from build123d import *

# Parameters (mm, degrees)
F1_DEPTH        = 25
F3_START        = -0.65
F2_R            = 4.3
F3_DEPTH        = 2.15
F3_COPIES_COUNT = 3
F6_DEPTH        = 23
F8_DEPTH        = 2
F9_SIZE         = 0.6
F10_SIZE        = 0.4


# Not quite as in the source:
# - a pattern or mirror of a feature is missing from the dataset's text; its kind, count and spacing are read off the source's solid


with BuildPart() as f1:
    # F0 (on Top) → F1 (new body)
    with BuildSketch(Plane.XY):
        with BuildLine():
            ThreePointArc((7.6794919243, -4), (19.8038475773, 3), (19.8038475773, 17))
            Line((19.8038475773, 17), (12.124355653, 30.3012701892))
            ThreePointArc((12.124355653, 30.3012701892), (0, 37.3012701892), (-12.124355653, 30.3012701892))
            Line((-12.124355653, 30.3012701892), (-19.8038475773, 17))
            ThreePointArc((-19.8038475773, 17), (-19.8038475773, 3), (-7.6794919243, -4))
            Line((-7.6794919243, -4), (0, -4))
            Line((0, -4), (7.6794919243, -4))
        make_face()
        with BuildLine():
            Line((7.6794919243, 0), (0, 0))
            Line((0, 0), (-7.6794919243, 0))
            ThreePointArc((-7.6794919243, 0), (-16.3397459622, 5), (-16.3397459622, 15))
            Line((-16.3397459622, 15), (-8.6602540378, 28.3012701892))
            ThreePointArc((-8.6602540378, 28.3012701892), (0, 33.3012701892), (8.6602540378, 28.3012701892))
            Line((8.6602540378, 28.3012701892), (16.3397459622, 15))
            ThreePointArc((16.3397459622, 15), (16.3397459622, 5), (7.6794919243, 0))
        make_face(mode=Mode.SUBTRACT)
    extrude(amount=F1_DEPTH)

    # F2 (on face) → F3 (cut)
    with BuildSketch(Plane(origin=(-22.2141016151, 12.8253175473, 0), x_dir=(-0.5, -0.8660254038, 0), z_dir=(-0.8660254038, 0.5, 0)).offset(F3_START)):
        with Locations((-12.5, 12.5)):
            Circle(F2_R)
    f3 = extrude(amount=-F3_DEPTH, mode=Mode.SUBTRACT)

    # F3_copies: F3 ×3 about axis
    f3_copies_axis = Axis((0, 14.433757, 0), (0, 0, 1))
    for i in range(1, F3_COPIES_COUNT):
        add(f3.rotate(f3_copies_axis, i * 360 / F3_COPIES_COUNT), mode=Mode.SUBTRACT)

    # F5 (on face) → F6 (cut)
    with BuildSketch(Plane(origin=(0, 0, 0), x_dir=(1, 0, 0), z_dir=(0, 0, -1))):
        with BuildLine():
            Line((9.6994845224, -28.9012701892), (17.3789764467, -15.6))
            ThreePointArc((17.3789764467, -15.6), (17.3789764467, -4.4), (7.6794919243, 1.2))
            Line((7.6794919243, 1.2), (-7.6794919243, 1.2))
            ThreePointArc((-7.6794919243, 1.2), (-17.3789764467, -4.4), (-17.3789764467, -15.6))
            Line((-17.3789764467, -15.6), (-9.6994845224, -28.9012701892))
            ThreePointArc((-9.6994845224, -28.9012701892), (0, -34.5012701892), (9.6994845224, -28.9012701892))
        make_face()
    extrude(amount=-F6_DEPTH, mode=Mode.SUBTRACT)

    # F7 (on face) → F8 (cut)
    with BuildSketch(Plane(origin=(0, 0, 0), x_dir=(1, 0, 0), z_dir=(0, 0, -1))):
        with BuildLine():
            Line((11.0851251684, -29.7012701892), (18.7646170928, -16.4))
            ThreePointArc((18.7646170928, -16.4), (18.7646170928, -3.6), (7.6794919243, 2.8))
            Line((7.6794919243, 2.8), (-7.6794919243, 2.8))
            ThreePointArc((-7.6794919243, 2.8), (-18.7646170928, -3.6), (-18.7646170928, -16.4))
            Line((-18.7646170928, -16.4), (-11.0851251684, -29.7012701892))
            ThreePointArc((-11.0851251684, -29.7012701892), (0, -36.1012701892), (11.0851251684, -29.7012701892))
        make_face()
    extrude(amount=-F8_DEPTH, mode=Mode.SUBTRACT)

    # F9
    f9_edges = [f1.edges().sort_by_distance(p)[0] for p in [
        (0, 34.50127, 2),
        (13.53923, 22.250635, 2),
        (17.378976, 4.4, 2),
        (0, -1.2, 2),
        (-17.378976, 4.4, 2),
        (-13.53923, 22.250635, 2),
    ]]
    chamfer(f9_edges, length=F9_SIZE)

    # F10
    f10_edges = [f1.edges().sort_by_distance(p)[0] for p in [
        (19.803848, 3, 25),
        (12.5, 21.650635, 25),
        (0, -4, 25),
        (-19.803848, 3, 25),
        (-15.964102, 23.650635, 25),
        (15.964102, 23.650635, 25),
        (0, 37.30127, 25),
        (16.339746, 5, 25),
        (0, 0, 25),
        (-16.339746, 5, 25),
        (-12.5, 21.650635, 25),
        (0, 33.30127, 25),
    ]]
    chamfer(f10_edges, length=F10_SIZE)


solid = f1.part
Check sheet for the modelled part. Datum: model origin and axes. Units: mm. A direction names the side the tool comes from. Coordinates: 2 decimals unless noted, no trailing zeros. Write each loop counter-clockwise with the first axis right and the second up, starting at its lowest first coordinate (ties: lowest second). Pieces come first, ordered by that corner, then holes. Notation, with made-up numbers: M 58,-0.5 L 90,-0.5 A16 cw 90,6.5 Z; hole C -38,35 d11. An arc over 180 degrees is marked long. Answer as CSV lines item,"result".
Q1. Cross-section at D-D (z = 11.75). Record the boundary of the cut face in (x, y), then the cut area to 3 significant figures.
Check result:
outline,"M -19.8,17 A14 ccw -7.68,-4 L 7.68,-4 A14 ccw 19.8,17 L 12.12,30.3 A14 ccw -12.12,30.3 Z; hole M -17.52,19.66 L -15.66,18.58 L -17.38,15.6 A11.2 ccw -7.68,-1.2 L -4.23,-1.2 L -4.23,-3.35 L 4.23,-3.35 L 4.23,-1.2 L 7.68,-1.2 A11.2 ccw 17.38,15.6 L 15.66,18.58 L 17.52,19.66 L 13.28,26.99 L 11.42,25.92 L 9.7,28.9 A11.2 ccw -9.7,28.9 L -11.42,25.92 L -13.28,26.99 Z"
area,"296 mm^2"
Q2. Mould release check, pull along X, two halves, no side actions. Record for faces 1 (the face through (-17.435, 4.175, 2.438)), 2 (the face through (15.84, 23.46, 24.8)), 3 (the face through (0, -1.2, 17)), 4 (the face through (-13, 23, 25)): released by +X, released by -X, zero draft, split by the parting line, or undercut.
Check result:
face 1,"undercut"
face 2,"released by +X"
face 3,"undercut"
face 4,"zero draft"
Q3. Set-up check for faces 5 (the face through (12.622, 21.845, 24.803)), 6 (the face through (-16.266, 4.874, 23.789)), 7 (the face through (-17.296, 4.258, 12.657)): record each of +Z, -Z, +X, -X, +Y, -Y from which the full face is reachable in a straight line by a thin tool's end or side.
Check result:
face 5,"+Z"
face 6,"+Z, -Z"
face 7,"-Z"
Q4. Go/stop test with flat-tipped pins: pin 1 (10 mm diameter, centred on y = 16.5, z = 20, fed in from -X); pin 2 (12 mm diameter, centred on y = 18.5, z = 7.5, fed in from +X); pin 3 (1 mm diameter, centred on y = 30.5, z = 21.5, fed in from +X). Record where each tip stops, or that it passes through.
Check result:
pin 1,"x = -21.6"
pin 2,"x = 21.45"
pin 3,"x = 12.3"
Q5. Cross-section at B-B (z = 21). Record the boundary of the cut face in (x, y), then the cut area to 3 significant figures.
Check result:
outline,"M -19.8,17 A14 ccw -7.68,-4 L 7.68,-4 A14 ccw 19.8,17 L 12.12,30.3 A14 ccw -12.12,30.3 Z; hole M -17.38,15.6 A11.2 ccw -7.68,-1.2 L 7.68,-1.2 A11.2 ccw 17.38,15.6 L 9.7,28.9 A11.2 ccw -9.7,28.9 Z"
area,"351 mm^2"
Q6. Cross-section at A-A (x = 0). Record the boundary of the cut face in (y, z), then the cut area to 3 significant figures.
Check result:
outline,"M -4,0 L -2.8,0 L -2.8,2 L -1.8,2 L -1.2,2.6 L -1.2,8.2 L -3.35,8.2 L -3.35,16.8 L -1.2,16.8 L -1.2,23 L 0,23 L 0,24.6 L -0.4,25 L -3.6,25 L -4,24.6 Z; M 33.3,23 L 34.5,23 L 34.5,2.6 L 35.1,2 L 36.1,2 L 36.1,0 L 37.3,0 L 37.3,24.6 L 36.9,25 L 33.7,25 L 33.3,24.6 Z"
area,"119 mm^2"
Q7. Cross-section at C-C (z = 15). Record the boundary of the cut face in (x, y).
Check result:
outline,"M -19.8,17 A14 ccw -7.68,-4 L 7.68,-4 A14 ccw 19.8,17 L 12.12,30.3 A14 ccw -12.12,30.3 Z; hole M -17.38,15.6 A11.2 ccw -7.68,-1.2 L -3.5,-1.2 L -3.5,-3.35 L 3.5,-3.35 L 3.5,-1.2 L 7.68,-1.2 A11.2 ccw 17.38,15.6 L 15.29,19.22 L 17.15,20.3 L 13.65,26.36 L 11.79,25.28 L 9.7,28.9 A11.2 ccw -9.7,28.9 L -11.79,25.28 L -13.65,26.36 L -17.15,20.3 L -15.29,19.22 Z"
Q8. Material ranges on probe 1 along Z at (x, y) = (0, -2.5); probe 2 along X at (y, z) = (26.5, 13.75); probe 3 along X at (y, z) = (9.5, 7), recorded low to high. Write a range as from..to.
Check result:
probe 1,"2..8.2, 16.8..25"
probe 2,"-14.32..-13.57, -12.67..-11.09, 11.09..12.67, 13.57..14.32"
probe 3,"-21.67..-18.87, 18.87..21.67"
